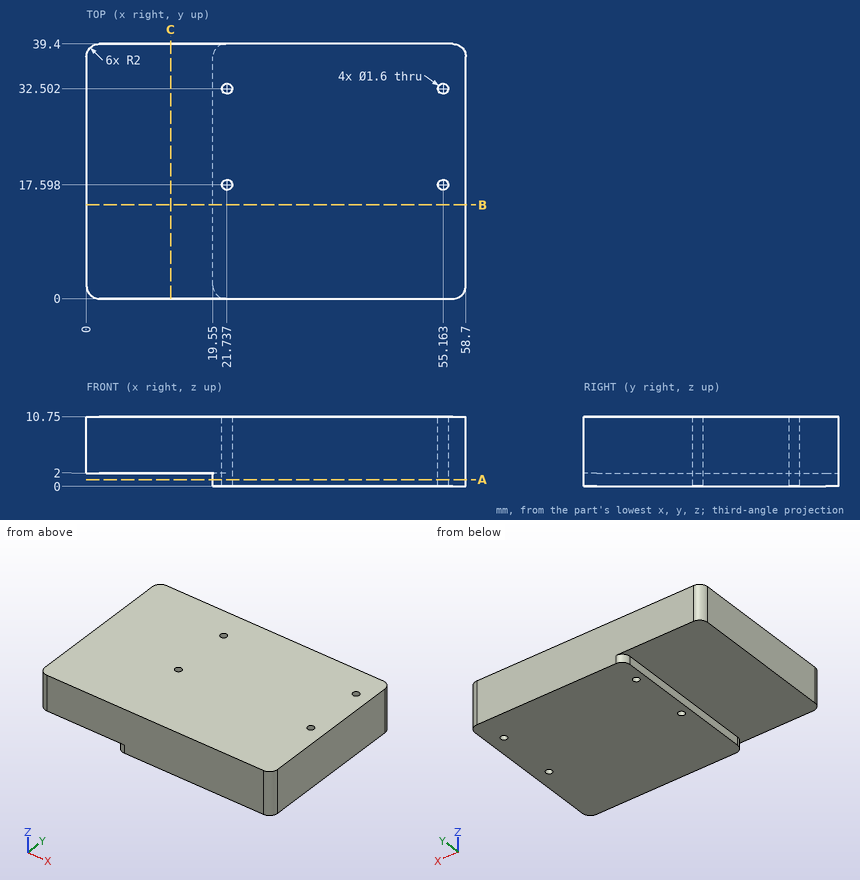
Can you work these out from the drawing? Everything is in mm from the part's minimum corner. Round coordinates to 2 decimals unless told otherwise and drop trailing zeros. Write each loop counter-clockwise with the first axis right and the second up, starting at its lowest first coordinate (ties: lowest second). Pieces come first, ordered by that corner, then holes. Notation, with made-up numbers: (51.25, -21.75) - (100.25, -21.75) arc R26 ccw to (100.25, 2.25) - close; hole circle Ø2 at (-30.75, 66.5). An arc over 180 degrees is marked (long way). Use a Markdown table: item, result.
Q1. I want a section at B-B (y = 14.5). List the corners of the cut face in (x, z) for me.
Output values:
| item | result |
|---|---|
| outline | (0, 2) - (19.55, 2) - (19.55, 0) - (58.7, 0) - (58.7, 10.75) - (0, 10.75) - close |
Q2. I want a section at A-A (z = 1). List the corners of the cut face in (x, y) for me.
Output values:
| item | result |
|---|---|
| outline | (19.55, 2) arc R2 ccw to (21.55, 0) - (56.7, 0) arc R2 ccw to (58.7, 2) - (58.7, 37.4) arc R2 ccw to (56.7, 39.4) - (21.55, 39.4) arc R2 ccw to (19.55, 37.4) - close; hole circle Ø1.6 at (21.74, 17.6); hole circle Ø1.6 at (21.74, 32.5); hole circle Ø1.6 at (55.16, 17.6); hole circle Ø1.6 at (55.16, 32.5) |
Q3. For pin 1 (5 mm diameter, centred on x = 6, y = 22.5, fed in from -Z); pin 2 (1.4 mm diameter, centred on x = 55.16, y = 17.6, fed in from +Z); pin 3 (2 mm diameter, centred on y = 26.5, z = 0.5, fed in from -X), each with a flat end and sliding along its axis, tell me the tip position at first contact or that it passes through.
Output values:
| item | result |
|---|---|
| pin 1 | z = 2 |
| pin 2 | through |
| pin 3 | x = 19.55 |
Q4. I want a section at C-C (x = 13). List the corners of the cut face in (y, z) for me.
Output values:
| item | result |
|---|---|
| outline | (0, 2) - (39.4, 2) - (39.4, 10.75) - (0, 10.75) - close |
Q5. Please list where these lines run through material, in increasing order: L1, parallel to X at y = 32.5, z = 9.5; L2, parallel to X at y = 18, z = 5.5 (1 decimal); L3, parallel to X at y = 36.5, z = 1.75.
Output values:
| item | result |
|---|---|
| L1 | 0 to 20.94, 22.54 to 54.36, 55.96 to 58.7 |
| L2 | 0 to 21, 22.4 to 54.5, 55.9 to 58.7 |
| L3 | 19.55 to 58.7 |
